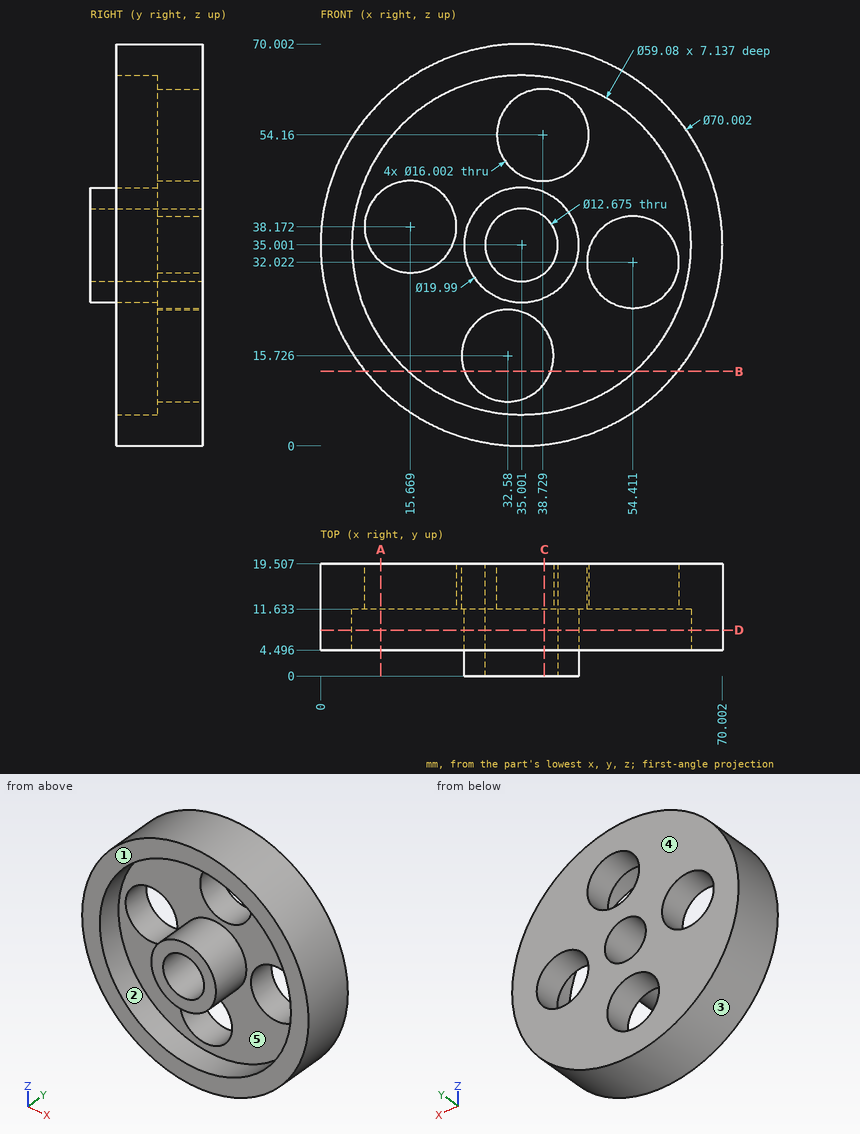
Drawing for the job (mm, zero at the part's lowest x, y, z). A direction names the side the tool comes from. Round coordinates to 2 decimals unless told otherwise and drop trailing zeros. Loops run counter-clockwise (first coordinate to the right, second up) from the corner with the lowest first, then second, coordinate; pieces in that order, holes last. Notation, with made-up numbers: (68, 83.25) - (73, 83.25) arc R29 ccw to (73, 104.25) - close; hole circle Ø3 at (83.5, 66). An arc over 180 degrees is marked (long way). Write each question's results on one line, items separated by ' | '.
(1) Wall check: L1, parallel to Z at x = 35.5, y = 16.5 (1 decimal); L2, parallel to Z at x = 31, y = 5 (1 decimal); L3, parallel to X at y = 9.75, z = 62 (1 decimal). Give the ranges that are in metal, low to high.
Answer below:
L1: z = 0 to 8.3, 23.2 to 28.7, 41.3 to 46.8, 61.5 to 70 | L2: z = 0.2 to 5.7, 25.8 to 30.1, 39.9 to 44.2, 64.3 to 69.8 | L3: x = 12.7 to 23, 47 to 57.3
(2) Saw through at D-D, the plane y = 8. List the corners of the cut face in (x, z) (1 decimal).
Answer below:
outline: circle Ø70 at (35, 35); circle Ø20 at (35, 35); hole circle Ø59.1 at (35, 35); hole circle Ø12.7 at (35, 35)
(3) 3-axis set-ups, long thin cutter, end or side, ignore diameter. For the marked faces 4 and 5: which of +Z, -Z, +X, -X, +Y, -Y reach the whole face in a straight line?
Answer below:
face 4: +Z, -Z, +X, -X, +Y | face 5: -Y
(4) Pin check, flat tips, straight feed: pin 1 (3 mm diameter, centred on y = 4, z = 14.5, fed in from -X); pin 2 (18.5 mm diameter, centred on x = 15.67, z = 38.17, fed in from -Y); pin 3 (3 mm diameter, centred on x = 23, y = 3.5, fed in from +Z). Stop position of each tip, or through.
Answer below:
pin 1: stops at x = 5.66 | pin 2: stops at y = 11.63 | pin 3: stops at z = 68.27
(5) Mould opens along X. For the marked faces 1, 2 and 3 say: released by +X, released by -X, zero draft, split by the parting line, or undercut.
Answer below:
face 1: zero draft | face 2: undercut | face 3: split by the parting line
(6) Saw through at A-A, the plane x = 10.5. List the corners of the cut face in (y, z) (1 decimal), then the cut area to 3 significant figures.
Answer below:
outline: (4.5, 10) - (19.5, 10) - (19.5, 32.1) - (11.6, 32.1) - (11.6, 18.5) - (4.5, 18.5) - close; (4.5, 51.5) - (11.6, 51.5) - (11.6, 44.3) - (19.5, 44.3) - (19.5, 60) - (4.5, 60) - close | area: 419 mm^2
(7) Saw through at C-C, the plane x = 39. List the corners of the cut face in (y, z) (1 decimal).
Answer below:
outline: (0, 25.8) - (11.6, 25.8) - (11.6, 20.5) - (19.5, 20.5) - (19.5, 30.1) - (0, 30.1) - close; (0, 39.9) - (19.5, 39.9) - (19.5, 46.2) - (11.6, 46.2) - (11.6, 44.2) - (0, 44.2) - close; (4.5, 0.2) - (19.5, 0.2) - (19.5, 11) - (11.6, 11) - (11.6, 5.7) - (4.5, 5.7) - close; (4.5, 64.3) - (11.6, 64.3) - (11.6, 62.2) - (19.5, 62.2) - (19.5, 69.8) - (4.5, 69.8) - close
(8) Saw through at B-B, the plane z = 13. List the corners of the cut face in (x, y) (1 decimal).
Answer below:
outline: (7.8, 4.5) - (15.3, 4.5) - (15.3, 11.6) - (25.1, 11.6) - (25.1, 19.5) - (7.8, 19.5) - close; (40.1, 11.6) - (54.7, 11.6) - (54.7, 4.5) - (62.2, 4.5) - (62.2, 19.5) - (40.1, 19.5) - close
